The model under review builds one solid part; all positions refer to its coordinate system, in mm. A direction names the side the tool comes from. Coordinates: 2 decimals unless noted, no trailing zeros. Order: outer loops, then holes, each group sorted by start corner. A loop starts at its lowest first (then second) coordinate and runs counter-clockwise, first axis right, second up.
from build123d import *

# Parameters (mm, degrees)
F0_W     = 129.5
F0_H     = 69.5
F1_DEPTH = 25
F2_T     = -2
F3_R     = 0.99999


# Not quite as in the source:
# - a fillet or chamfer is up to 0.001 mm smaller than in the source, because OpenCascade refuses the exact size


with BuildPart() as f1:
    # F0 (on Top) → F1 (new body)
    with BuildSketch(Plane.XY):
        with Locations((8.1922735609, -6.6703366488)):
            Rectangle(F0_W, F0_H)
    extrude(amount=F1_DEPTH)

    # F2
    f2_openings = [f1.faces().sort_by_distance(p)[0] for p in [
        (8.192274, -6.670337, 25),
    ]]
    offset(amount=F2_T, openings=f2_openings)

    # F3 (radius 1 in the source; OpenCascade refuses exactly that, so slightly less here)
    f3_edges = [f1.edges().sort_by_distance(p)[0] for p in [
        (8.192274, 26.079663, 25),
        (-56.557726, -6.670337, 25),
        (-54.557726, -6.670337, 25),
        (8.192274, -41.420337, 25),
        (72.942274, -6.670337, 0),
        (72.942274, -6.670337, 25),
        (8.192274, -39.420337, 25),
        (8.192274, 28.079663, 25),
        (72.942274, 28.079663, 12.5),
        (-56.557726, 28.079663, 12.5),
        (-56.557726, -41.420337, 12.5),
        (-54.557726, 26.079663, 13.5),
        (72.942274, -41.420337, 12.5),
    ]]
    fillet(f3_edges, radius=F3_R)


solid = f1.part
(1) Wall thickness on line 1 (Y direction, x = -36.5, z = 9); line 2 (X direction, y = 2.5, z = 19); line 3 (Z direction, x = -0.5, y = 5.5): over which ranges is each line inside the solid? List them lowest first.
(2) The part is to be moulded in two halves that separate along X. For faces 3 (the face through (8, 26.08, 13)), 4 (the face through (7, -6, 0)), 5 (the face through (72.942, -7, 12)), 6 (the face through (7, -39.42, 13)), say which applies: +X half, -X half, draft (parallel to the pull), parting line (faces both ways), or undercut.
(3) Tool access review of faces 1 (the face through (7, -41.42, 12)), 2 (the face through (-54.558, -8, 13)): name each direction out of +Z, -Z, +X, -X, +Y, -Y from which nothing blocks a thin tool from reaching the whole face with its end or side.
(4) Consider section A-A (z = 13). Give the boundary of the cut face in (x, y), then the cut area to 3 significant figures.
(5) Insertion check: pin 1 Ø2 at (x, y) = (6.5, -18) entering from +Z. The pin has a flat end and moves straight along its axis. Give the tip position at first contact, or say it passes through.
Findings:
1. line 1: y = -41.42 to -39.42, 26.08 to 28.08
1. line 2: x = -56.56 to -54.56, 70.94 to 72.94
1. line 3: z = 0 to 2
2. face 3: undercut
2. face 4: draft
2. face 5: +X half
2. face 6: undercut
3. face 1: +Z, -Z, +X, -X, -Y
3. face 2: +Z
4. outline: (-56.56, -40.42) arc R1 ccw to (-55.56, -41.42) - (71.94, -41.42) arc R1 ccw to (72.94, -40.42) - (72.94, 27.08) arc R1 ccw to (71.94, 28.08) - (-55.56, 28.08) arc R1 ccw to (-56.56, 27.08) - close; hole (-54.56, -39.42) - (70.94, -39.42) - (70.94, 26.08) - (-53.56, 26.08) arc R1 ccw to (-54.56, 25.08) - close
4. area: 779 mm2
5. pin 1: stops at z = 2
